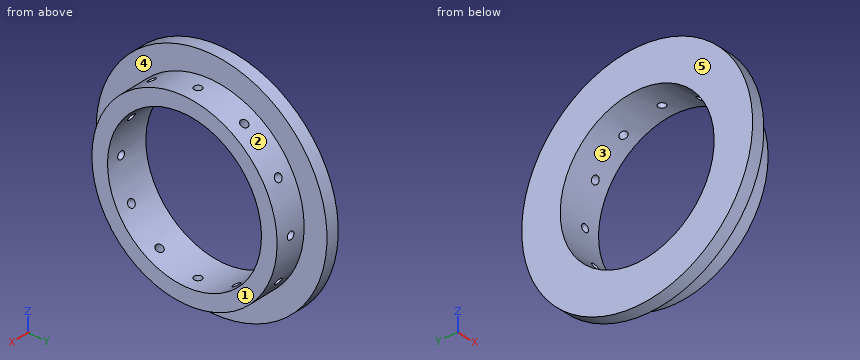
from build123d import *

# Parameters (mm, degrees)
SKETCH1_R           = 57.15
SKETCH1_R_2         = 38.1
BOSS_EXTRUDE1_DEPTH = 6.35
SKETCH2_R           = 45.847
SKETCH2_R_2         = 38.1
BOSS_EXTRUDE2_DEPTH = 15.24
SKETCH4_R           = 1.89865
CUT_EXTRUDE1_DEPTH  = 11.43
CIRPATTERN1_COUNT   = 12


with BuildPart() as part:
    # Sketch1 → Boss-Extrude1 (new body)
    with BuildSketch(Plane(origin=(0, 0, 0), x_dir=(0, 0, -1), z_dir=(1, 0, 0))):
        Circle(SKETCH1_R)
        Circle(SKETCH1_R_2, mode=Mode.SUBTRACT)
    extrude(amount=BOSS_EXTRUDE1_DEPTH)

    # Sketch2 → Boss-Extrude2 (add)
    with BuildSketch(Plane(origin=(6.35, 0, 0), x_dir=(0, 0, -1), z_dir=(1, 0, 0))):
        Circle(SKETCH2_R)
        Circle(SKETCH2_R_2, mode=Mode.SUBTRACT)
    extrude(amount=BOSS_EXTRUDE2_DEPTH)

    # Sketch4 → Cut-Extrude1 (cut)
    with BuildSketch(Plane(origin=(0, 0, -45.847), x_dir=(-1, 0, 0), z_dir=(0, 0, -1))):
        with Locations((-13.97, 0)):
            Circle(SKETCH4_R)
    cut_extrude1 = extrude(amount=-CUT_EXTRUDE1_DEPTH, mode=Mode.SUBTRACT)

    # CirPattern1: Cut-Extrude1 ×12 about axis
    cirpattern1_axis = Axis((0, 0, 0), (1, 0, 0))
    for i in range(1, CIRPATTERN1_COUNT):
        add(cut_extrude1.rotate(cirpattern1_axis, i * 360 / CIRPATTERN1_COUNT), mode=Mode.SUBTRACT)


solid = part.part
Work out the finished part from the listing and answer in its coordinate system (mm). Face numbers are marked on the shaded views. A direction names the side the tool comes from. Give positions to 0.01 mm unless a question says otherwise; leave off trailing zeros. Loops run counter-clockwise (first coordinate to the right, second up) from the corner with the lowest first, then second, coordinate; pieces in that order, holes last. Notation, with made-up numbers: (-15.5, -5.75) -> (29.5, -5.75) arc R13 cw to (29.5, 3.25) -> close; hole circle Ø9 at (62, 17). An arc over 180 degrees is marked (long way). Use a Markdown table: item, result. Add a question column.
1. For the marked faces 4 and 5, determine the directions among +Z, -Z, +X, -X, +Y, -Y from which every point of the face is accessible in a straight line to the end or side of a thin tool.
2. Flat-ended cylindrical pins translate along their axes: pin 1 Ø4 at (x, z) = (13, 7) entering from -Y; pin 2 Ø10 at (x, z) = (7, -28.5) entering from -Y; pin 3 Ø4.5 at (x, y) = (13.97, 0) entering from +Z. Find the tip coordinate at first contact, or state that the pin passes through.
3. Determine the mould class of the marked faces 1, 2 and 3 for opening direction Z: released by +Z, released by -Z, zero draft, split by the parting line, or undercut.
4. Section A-A on y = 0 is taken. Determine the outline of the cut face in (x, z), and give its area (3 significant figures).
5. Find the intervals of material crossed by probe 1 along Z at (x, y) = (2.75, -0.5); probe 2 along X at (y, z) = (40.75, 0); probe 3 along X at (y, z) = (-46, -30.5), in increasing order.
6. Section D-D on y = 26 is taken. Determine the outline of the cut face in (x, z).
7. Section C-C on x = 2.75 is taken. Determine the outline of the cut face in (y, z).
Results below:
| question | item | result |
|---|---|---|
| 1 | face 4 | +X |
| 1 | face 5 | +Z, -Z, -X, +Y, -Y |
| 2 | pin 1 | stops at y = -45.57 |
| 2 | pin 2 | stops at y = -52.08 |
| 2 | pin 3 | stops at z = 45.85 |
| 3 | face 1 | zero draft |
| 3 | face 2 | split by the parting line |
| 3 | face 3 | undercut |
| 4 | outline | (0, -57.15) -> (6.35, -57.15) -> (6.35, -45.85) -> (12.07, -45.85) -> (12.07, -38.1) -> (0, -38.1) -> close; (0, 38.1) -> (12.07, 38.1) -> (12.07, 45.85) -> (6.35, 45.85) -> (6.35, 57.15) -> (0, 57.15) -> close; (15.87, -45.85) -> (21.59, -45.85) -> (21.59, -38.1) -> (15.87, -38.1) -> close; (15.87, 38.1) -> (21.59, 38.1) -> (21.59, 45.85) -> (15.87, 45.85) -> close |
| 4 | area | 419 mm^2 |
| 5 | probe 1 | z = -57.15 to -38.1, 38.1 to 57.15 |
| 5 | probe 2 | x = 0 to 12.07, 15.87 to 21.59 |
| 5 | probe 3 | x = 0 to 6.35 |
| 6 | outline | (0, -50.89) -> (6.35, -50.89) -> (6.35, -37.76) -> (21.59, -37.76) -> (21.59, -27.85) -> (0, -27.85) -> close; (0, 27.85) -> (21.59, 27.85) -> (21.59, 37.76) -> (6.35, 37.76) -> (6.35, 50.89) -> (0, 50.89) -> close |
| 7 | outline | circle Ø114.3 at (0, 0); hole circle Ø76.2 at (0, 0) |
